CAD build for the part. Positions are in the model's coordinates, mm. Coordinates: 2 decimals unless noted, no trailing zeros. Write each question's results on one line, items separated by ' | '.
```python
from build123d import *

# Parameters (mm, degrees)
CYLINDER129_R             = 1.75
CYLINDER129_DEPTH         = 26
CYLINDER131_R             = 1.75
CYLINDER131_DEPTH         = 26
BOX066_W                  = 7
BOX066_H                  = 48
BOX066_DEPTH              = 1
CYLINDER132_R             = 1.5
CYLINDER132_DEPTH         = 10
CYLINDER130_R             = 5
CYLINDER130_DEPTH         = 1
CYLINDER128_R             = 17.5
CYLINDER128_DEPTH         = 22
FUSION092_ROLL_ANGLE      = 90.000203
FUSION092_PITCH_ANGLE     = -15.000283
FUSION092_PLACEMENT_ANGLE = 90.000203


with BuildPart() as cylinder129:
    # Cylinder129 → Cylinder129 (new body)
    with BuildSketch(Plane(origin=(0, 21, 0), x_dir=(1, 0, 0), z_dir=(0, 0, 1))):
        Circle(CYLINDER129_R)
    extrude(amount=CYLINDER129_DEPTH)


with BuildPart() as cylinder131:
    # Cylinder131 → Cylinder131 (new body)
    with BuildSketch(Plane(origin=(0, -21, 0), x_dir=(1, 0, 0), z_dir=(0, 0, 1))):
        Circle(CYLINDER131_R)
    extrude(amount=CYLINDER131_DEPTH)


with BuildPart() as cut183:
    # Box066 → Box066 (new body)
    with BuildSketch(Plane(origin=(-3.4, -23.6, 22), x_dir=(1, 0, 0), z_dir=(0, 0, 1))):
        with Locations((3.5, 24)):
            Rectangle(BOX066_W, BOX066_H)
    extrude(amount=BOX066_DEPTH)

    # Cut182: cut Cylinder131
    add(cylinder131.part, mode=Mode.SUBTRACT)

    # Cut183: cut Cylinder129
    add(cylinder129.part, mode=Mode.SUBTRACT)


with BuildPart() as cut183_1:
    # Cut183 placement: moved
    add(cut183.part.moved(Location((0, 0, -1))))


with BuildPart() as cylinder132:
    # Cylinder132 → Cylinder132 (new body)
    with BuildSketch(Plane.XY.offset(23)):
        Circle(CYLINDER132_R)
    extrude(amount=CYLINDER132_DEPTH)


with BuildPart() as cylinder130:
    # Cylinder130 → Cylinder130 (new body)
    with BuildSketch(Plane.XY.offset(22)):
        Circle(CYLINDER130_R)
    extrude(amount=CYLINDER130_DEPTH)


with BuildPart() as fusion092:
    # Cylinder128 → Cylinder128 (new body)
    with BuildSketch(Plane.XY):
        Circle(CYLINDER128_R)
    extrude(amount=CYLINDER128_DEPTH)

    # Fusion092: union Cut183, Cylinder132, Cylinder130
    add(cut183_1.part)
    add(cylinder132.part)
    add(cylinder130.part)


with BuildPart() as fusion092_1:
    # Fusion092 roll: moved
    add(fusion092.part.rotate(Axis((0, 0, 0), (1, 0, 0)), FUSION092_ROLL_ANGLE))


with BuildPart() as fusion092_2:
    # Fusion092 pitch: moved
    add(fusion092_1.part.rotate(Axis((0, 0, 0), (0, 1, 0)), FUSION092_PITCH_ANGLE))


with BuildPart() as fusion092_3:
    # Fusion092 placement: moved
    add(fusion092_2.part.moved(Location((72.9, 55.9, 45.7))).rotate(Axis((72.9, 55.9, 45.7), (0, 0, 1)), FUSION092_PLACEMENT_ANGLE))


solid = fusion092_3.part
```
Q1. Pull direction Z, two halves, no side cores. Call faces 1 (the cylindrical face through (94.393, 51.647, 64.694)), 2 (the cylindrical face through (100.83, 54.436, 45.376)): +Z half, -Z half, draft (parallel to the pull), parting line (faces both ways), or undercut.
Results are:
face 1: undercut | face 2: parting line
Q2. Drop flat-ended pins along their axis: pin 1 (1.5 mm diameter, centred on x = 95, y = 64, fed in from +Z); pin 2 (3 mm diameter, centred on y = 50.46, z = 65.98, fed in from -X); pin 3 (12 mm diameter, centred on x = 78, z = 38, fed in from -Y); pin 4 (6 mm diameter, centred on y = 60.5, z = 47.5, fed in from +X). Give the stop position or say it passes through.
Results are:
pin 1: z = 61.58 | pin 2: through | pin 3: y = 38.48 | pin 4: x = 95.9
Q3. Wall check: L1, parallel to X at y = 62.5, z = 43; L2, parallel to Y at x = 94.5, z = 27; L3, parallel to X at y = 53.5, z = 43. Give the ranges that are in metal, low to high. Write a range as from..to.
Results are:
L1: 72.9..94.9 | L2: 57.39..60.59, 62.08..64.64 | L3: 72.9..95.9
